```python
from build123d import *

# Parameters (mm, degrees)
F0_W     = 330.2
F0_H     = 254
F1_DEPTH = 6.35
F3_D     = 12.7
F5_D     = 15.875
F7_D     = 9.525


with BuildPart() as f1:
    # F0 (on Top) → F1 (new body, symmetric)
    with BuildSketch(Plane.XY):
        Rectangle(F0_W, F0_H)
    extrude(amount=F1_DEPTH, both=True)

    # F3 (through all)
    with Locations(Plane.XY.offset(6.35)):
        with Locations((0, 22.225), (0, -22.225)):
            Hole(F3_D / 2)

    # F5 (through all)
    with Locations(Plane.XY.offset(6.35)):
        with Locations((0, 0)):
            Hole(F5_D / 2)

    # F7 (through all)
    with Locations(Plane.XY.offset(6.35)):
        with Locations((-69.85, 42.8625), (-139.7, 42.8625), (-139.7, -42.8625), (-69.85, -42.8625), (69.85, 42.8625), (139.7, 42.8625), (139.7, -42.8625), (69.85, -42.8625)):
            Hole(F7_D / 2)


solid = f1.part
```
Verification items for the finished model (mm, model axes). Round coordinates to 2 decimals unless told otherwise and drop trailing zeros. Write each loop counter-clockwise with the first axis right and the second up, starting at its lowest first coordinate (ties: lowest second). Pieces come first, ordered by that corner, then holes.
1. Section check A-A on y = 0. Enter the section's corners in (x, z).
2. Scan lines: L1, parallel to Y at x = -69.85, z = 0 (3 decimals); L2, parallel to X at y = 1, z = -3; L3, parallel to Y at x = 71, z = -2.75. Record each from-to range of solid material in increasing order.
3. Gauge pin test, flat end, axial feed: P1, Ø8.5, axis at x = 139.7, y = 42.86, coming from the +Z side. Record the tip position at first contact, or that the pin passes through.
4. Draft check along Y on faces 1 (the flat face through (-165.1, -2, 0)), 2 (the cylindrical face through (-72.048, -47.088, -0.089)), 3 (the flat face through (-2, -127, 0)), 4 (the cylindrical face through (67.29, 46.88, -0.09)). Enter one of: +Y half, -Y half, draft (parallel to the pull), parting line (faces both ways), or undercut.
5. Section check B-B on x = 139.7. Enter the section's corners in (y, z) (3 decimals).
Answer:
1. outline: (-165.1, -6.35) - (-7.94, -6.35) - (-7.94, 6.35) - (-165.1, 6.35) - close; (7.94, -6.35) - (165.1, -6.35) - (165.1, 6.35) - (7.94, 6.35) - close
2. L1: y = -127 to -47.625, -38.1 to 38.1, 47.625 to 127
2. L2: x = -165.1 to -7.87, 7.87 to 165.1
2. L3: y = -127 to -47.48, -38.24 to 38.24, 47.48 to 127
3. P1: passes through
4. face 1: draft
4. face 2: undercut
4. face 3: -Y half
4. face 4: undercut
5. outline: (-127, -6.35) - (-47.625, -6.35) - (-47.625, 6.35) - (-127, 6.35) - close; (-38.1, -6.35) - (38.1, -6.35) - (38.1, 6.35) - (-38.1, 6.35) - close; (47.625, -6.35) - (127, -6.35) - (127, 6.35) - (47.625, 6.35) - close
